Work out the finished part from the listing and answer in its coordinate system (mm). Give positions to 0.01 mm unless a question says otherwise; leave off trailing zeros. Order: outer loops, then holes, each group sorted by start corner. A loop starts at its lowest first (then second) coordinate and runs counter-clockwise, first axis right, second up. Notation, with made-up numbers: (-11, -37) -> (42, -37) arc R35 cw to (42, 1) -> close; hole circle Ø6 at (61.5, 43.5). An arc over 180 degrees is marked (long way). Answer as CSV lines item,"result". Start each with the question number.
1. A cutting plane is placed at B-B (z = -22.5). Give the vertices of the cut face in (x, y).
2. A cutting plane is placed at C-C (x = 2.1). Give the vertices of the cut face in (y, z), then the cut area to 3 significant figures.
3. A cutting plane is placed at A-A (z = -10). Give the vertices of the cut face in (x, y).
4. Find the intervals of material crossed by L1, parallel to Y at x = 1.55, z = 22.5; L2, parallel to Y at x = 1.9, z = 10; L3, parallel to Z at x = 1.2, y = -1, in increasing order.
5. Flat-ended cylindrical pins translate along their axes: pin 1 (2.5 mm diameter, centred on y = 0, z = -10, fed in from -X); pin 2 (1.5 mm diameter, centred on x = 1.5, y = -4, fed in from -Z). Find the tip coordinate at first contact, or state that the pin passes through.
6. A cutting plane is placed at D-D (y = -11). Give the vertices of the cut face in (x, z).
from build123d import *

# Parameters (mm, degrees)
SKETCH_1_W          = 60
SKETCH_1_H          = 40
EXTRUDE_1_DEPTH     = 3
SKETCH_2_R          = 1.51
CUT_EXTRUDE_1_DEPTH = 10
SKETCH_3_R          = 1.51
CUT_EXTRUDE_2_DEPTH = 10
CUT_EXTRUDE_3_DEPTH = 10
FILLET_1_R          = 2


with BuildPart() as part:
    # 草图1 → 凸台-拉伸1 (new body)
    with BuildSketch(Plane(origin=(0, 0, 0), x_dir=(0, 0, -1), z_dir=(1, 0, 0))):
        Rectangle(SKETCH_1_W, SKETCH_1_H)
    extrude(amount=EXTRUDE_1_DEPTH)

    # 草图2 → 切除-拉伸1 (cut)
    with BuildSketch(Plane.ZY):
        with Locations((-22.5, -11)):
            Circle(SKETCH_2_R)
        with Locations((22.5, -11)):
            Circle(SKETCH_2_R)
        with Locations((22.5, 11)):
            Circle(SKETCH_2_R)
        with Locations((-22.5, 11)):
            Circle(SKETCH_2_R)
    extrude(amount=-CUT_EXTRUDE_1_DEPTH, mode=Mode.SUBTRACT)

    # 草图3 → 切除-拉伸2 (cut)
    with BuildSketch(Plane.ZY):
        with Locations((10, 0)):
            Circle(SKETCH_3_R)
        with Locations((-10, 0)):
            Circle(SKETCH_3_R)
    extrude(amount=-CUT_EXTRUDE_2_DEPTH, mode=Mode.SUBTRACT)

    # 草图4 → 切除-拉伸3 (cut)
    with BuildSketch(Plane(origin=(3, 0, 0), x_dir=(0, 0, -1), z_dir=(1, 0, 0))):
        Polygon((26, -7), (30, -11), (30, 3), (26, -1), align=None)
    extrude(amount=-CUT_EXTRUDE_3_DEPTH, mode=Mode.SUBTRACT)

    # 圆角1
    fillet_1_edges = [part.edges().sort_by_distance(p)[0] for p in [
        (1.5, -1, -26),
        (1.5, 3, -30),
        (1.5, -11, -30),
        (1.5, -7, -26),
        (1.5, -20, -30),
        (1.5, -20, 30),
        (1.5, 20, 30),
        (1.5, 20, -30),
    ]]
    fillet(fillet_1_edges, radius=FILLET_1_R)


solid = part.part
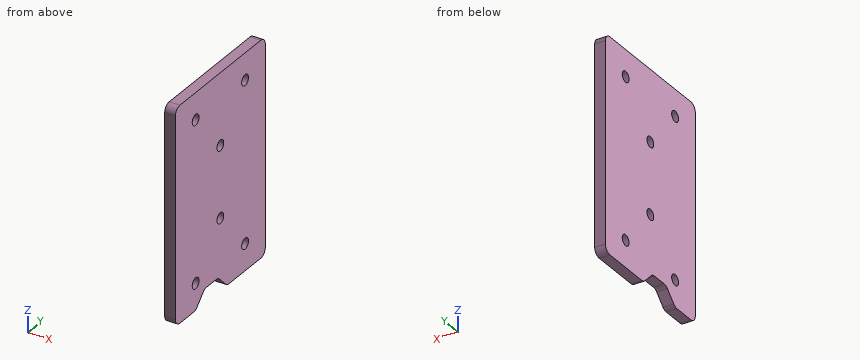
Answer sheet:
1,outline,"(0, -20) -> (3, -20) -> (3, -12.51) -> (0, -12.51) -> close; (0, -9.49) -> (3, -9.49) -> (3, 9.49) -> (0, 9.49) -> close; (0, 12.51) -> (3, 12.51) -> (3, 20) -> (0, 20) -> close"
2,outline,"(-20, -28) arc R2 ccw to (-18, -30) -> (-11.83, -30) arc R2 ccw to (-10.41, -29.41) -> (-7.59, -26.59) arc R2 cw to (-6.17, -26) -> (-1.83, -26) arc R2 cw to (-0.41, -26.59) -> (2.41, -29.41) arc R2 ccw to (3.83, -30) -> (18, -30) arc R2 ccw to (20, -28) -> (20, 28) arc R2 ccw to (18, 30) -> (-18, 30) arc R2 ccw to (-20, 28) -> close; hole circle Ø3.02 at (-11, -22.5); hole circle Ø3.02 at (-11, 22.5); hole circle Ø3.02 at (0, -10); hole circle Ø3.02 at (0, 10); hole circle Ø3.02 at (11, -22.5); hole circle Ø3.02 at (11, 22.5)"
2,area,"2,310 mm^2"
3,outline,"(0, -20) -> (3, -20) -> (3, -1.51) -> (0, -1.51) -> close; (0, 1.51) -> (3, 1.51) -> (3, 20) -> (0, 20) -> close"
4,L1,"y = -20 to -12.51, -9.49 to 9.49, 12.51 to 20"
4,L2,"y = -20 to -1.51, 1.51 to 20"
4,L3,"z = -26.18 to -11.13, -8.87 to 8.87, 11.13 to 30"
5,pin 1,"passes through"
5,pin 2,"stops at z = -26"
6,outline,"(0, -29.82) -> (3, -29.82) -> (3, -24.01) -> (0, -24.01) -> close; (0, -20.99) -> (3, -20.99) -> (3, 20.99) -> (0, 20.99) -> close; (0, 24.01) -> (3, 24.01) -> (3, 30) -> (0, 30) -> close"
